from build123d import *

# Parameters (mm, degrees)
F0_W     = 203.2
F0_H     = 158.75
F1_DEPTH = 25.4
F2_W     = 25.4
F2_H     = 127
F3_DEPTH = 25.4
F4_R     = 6.35
F5_DEPTH = 177.8
F6_R     = 6.35
F7_DEPTH = 177.8
F8_W     = 101.6
F8_H     = 127
F9_DEPTH = 25.4


with BuildPart() as f1:
    # F0 (on Front) → F1 (new body)
    with BuildSketch(Plane.XZ):
        with Locations((6.657936, 27.667538)):
            Rectangle(F0_W, F0_H)
    extrude(amount=F1_DEPTH)

    # F2 (on face) → F3 (cut)
    with BuildSketch(Plane.XZ.offset(25.4)):
        with Locations((-82.242064, 30.842538)):
            Rectangle(F2_W, F2_H)
        with Locations((95.557936, 30.842538)):
            Rectangle(F2_W, F2_H)
    extrude(amount=-F3_DEPTH, mode=Mode.SUBTRACT)

    # F4 (on face) → F5 (cut)
    with BuildSketch(Plane(origin=(0, 0, -51.707462), x_dir=(1, 0, 0), z_dir=(0, 0, -1))):
        with Locations((-44.142064, 12.7)):
            Circle(F4_R)
        with Locations((57.457936, 12.7)):
            Circle(F4_R)
    extrude(amount=-F5_DEPTH, mode=Mode.SUBTRACT)

    # F6 (on face) → F7 (cut)
    with BuildSketch(Plane(origin=(0, 0, -51.707462), x_dir=(1, 0, 0), z_dir=(0, 0, -1))):
        with Locations((-82.242064, 12.7)):
            Circle(F6_R)
        with Locations((95.557936, 12.7)):
            Circle(F6_R)
    extrude(amount=-F7_DEPTH, mode=Mode.SUBTRACT)

    # F8 (on face) → F9 (cut)
    with BuildSketch(Plane.XZ.offset(25.4)):
        with Locations((6.657936, 30.842538)):
            Rectangle(F8_W, F8_H)
    extrude(amount=-F9_DEPTH, mode=Mode.SUBTRACT)


solid = f1.part
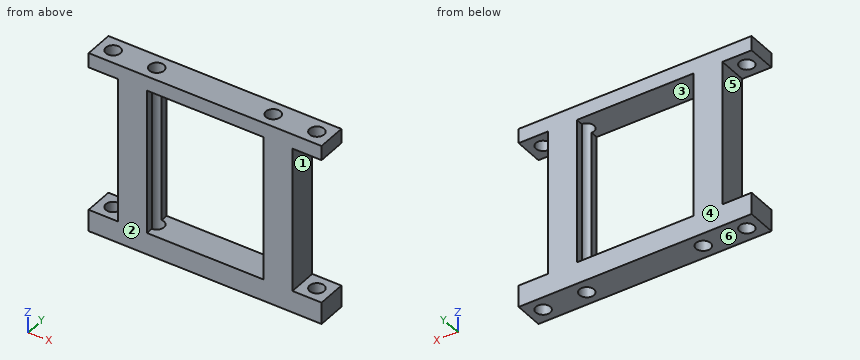
Check sheet for the modelled part. Datum: model origin and axes. Units: mm. Face numbers are marked on the shaded views. A direction names the side the tool comes from. Coordinates: 2 decimals unless noted, no trailing zeros. Loops run counter-clockwise (first coordinate to the right, second up) from the corner with the lowest first, then second, coordinate; pieces in that order, holes last. Notation, with made-up numbers: (44, -5) -> (51, -5) arc R19 ccw to (51, 13) -> close; hole circle Ø2 at (21, 50.5). An arc over 180 degrees is marked (long way). Answer in a Markdown table with one row per item.
1. Sectioned sample at A-A, the plane z = -18.5. Record the boundary of the cut face in (x, y), then the cut area to 3 significant figures.
Check values:
| item | result |
|---|---|
| outline | (-69.54, -25.4) -> (-44.14, -25.4) -> (-44.14, -19.05) arc R6.35 cw to (-44.14, -6.35) -> (-44.14, 0) -> (-69.54, 0) -> close; (57.46, -25.4) -> (82.86, -25.4) -> (82.86, 0) -> (57.46, 0) -> (57.46, -6.35) arc R6.35 cw to (57.46, -19.05) -> close |
| area | 1,160 mm2 |
2. Release check for a two-part mould opening along Z. For the marked faces 4, 5 and 6 record: released by +Z, released by -Z, zero draft, split by the parting line, or undercut.
Check values:
| item | result |
|---|---|
| face 4 | zero draft |
| face 5 | undercut |
| face 6 | released by -Z |
3. Sectioned sample at B-B, the plane x = 5. Record the boundary of the cut face in (y, z), then the cut area to 3 significant figures.
Check values:
| item | result |
|---|---|
| outline | (-25.4, -51.71) -> (0, -51.71) -> (0, -32.66) -> (-25.4, -32.66) -> close; (-25.4, 94.34) -> (0, 94.34) -> (0, 107.04) -> (-25.4, 107.04) -> close |
| area | 806 mm2 |
4. Access from +Z, -Z, +X, -X, +Y, -Y to the whole of each face (thin tool, end or side, straight path). Record for the marked faces 1, 2 and 3.
Check values:
| item | result |
|---|---|
| face 1 | +X, +Y, -Y |
| face 2 | +Z, -Z, +X, -X, -Y |
| face 3 | +Y, -Y |
5. Go/stop test with flat-tipped pins: pin 1 (7 mm diameter, centred on y = -4, z = 2.5, fed in from -X); pin 2 (10 mm diameter, centred on y = -6.5, z = 15, fed in from +X). Record where each tip stops, or that it passes through.
Check values:
| item | result |
|---|---|
| pin 1 | stops at x = -69.54 |
| pin 2 | stops at x = 82.86 |
6. Material ranges on line 1 along X through (y, z) = (-12.7, 103.75); line 2 along Z through (x, y) = (31.5, -13.25); line 3 along X through (y, z) = (-23, 6), recorded low to high. Write a range as [from, to].
Check values:
| item | result |
|---|---|
| line 1 | x = [-94.94, -88.59], [-75.89, -50.49], [-37.79, 51.11], [63.81, 89.21], [101.91, 108.26] |
| line 2 | z = [-51.71, -32.66], [94.34, 107.04] |
| line 3 | x = [-69.54, -44.14], [57.46, 82.86] |
7. Sectioned sample at C-C, the plane y = -12.7. Give the number of separate pieces and of enclosed holes in the cut face, then the cut area to 3 significant figures.
Check values:
| item | result |
|---|---|
| separate pieces | 8 |
| enclosed holes | 0 |
| area | 9,680 mm2 |
